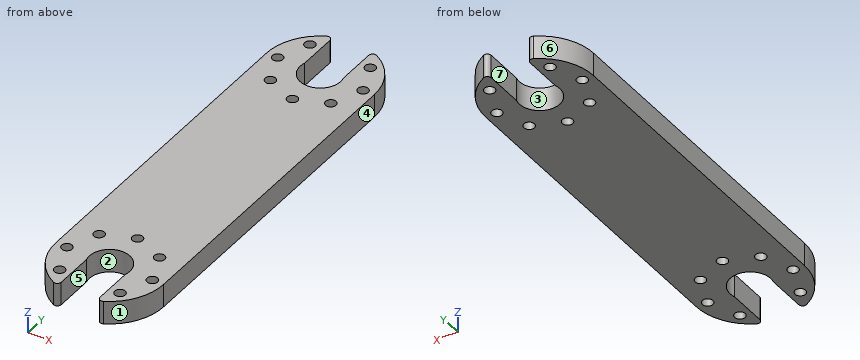
Autodesk Inventor part; units mm, degrees
ref_plane "YZ Plane" through (0, 0, 0) normal (1, 0, 0) x (0, 1, 0)
ref_plane "XZ Plane" through (0, 0, 0) normal (0, 1, 0) x (-1, 0, 0)
ref_plane "XY Plane" through (0, 0, 0) normal (0, 0, 1) x (1, 0, 0)
sketch "스케치1" plane through (0, 0, 0) normal (0, 0, 1) x (1, 0, 0)
  circle A0 centre (4.8832, 36.8726) radius 5
  circle A1 centre (4.8832, 47.8726) radius 1.55
  circle A2 centre (4.8832, 36.8726) radius 5
  arc A3 (-0.1168, 38.3009) -> (9.8832, 38.3009) centre (4.8832, 36.8726) ccw
  line L0 (4.8832, 42.0726) -> (9.8832, 42.0726)
  line L1 (4.8832, 42.0726) -> (-0.1168, 42.0726)
  circle A4 centre (4.8832, 36.8726) radius 13.9
  line L2 (9.8832, 42.0726) -> (9.8832, 49.8422)
  line L3 (-0.1168, 42.0726) -> (-0.1168, 49.8422)
  line L4 (9.8832, 42.0726) -> (9.8832, 38.3009)
  line L5 (-0.1168, 42.0726) -> (-0.1168, 38.3009)
  circle A5 centre (4.8832, 36.8726) radius 1.5
  line L6 (18.7832, 36.8726) -> (18.7832, -4.6274)
  line L7 (-9.0168, 36.8726) -> (-9.0168, -4.6274)
  arc A6 (-0.1168, 49.8422) -> (-9.0168, 36.8726) centre (4.8832, 36.8726) ccw
  arc A7 (18.7832, 36.8726) -> (9.8832, 49.8422) centre (4.8832, 36.8726) ccw
  line L8 (-9.0168, -4.6274) -> (18.7832, -4.6274)
  circle A8 centre (4.8832, 36.8726) radius 13.9
  line L9 (-9.0168, -46.1274) -> (-9.0168, -4.6274)
  line L10 (18.7832, -46.1274) -> (18.7832, -4.6274)
  line L11 (18.7832, -4.6274) -> (-9.0168, -4.6274)
  circle A9 centre (-2.895, 44.6508) radius 1.35
  circle A10 centre (-6.1168, 36.8726) radius 1.35
  circle A11 centre (-2.895, 29.0945) radius 1.35
  circle A12 centre (4.8832, 25.8726) radius 1.35
  circle A13 centre (12.6614, 29.0945) radius 1.35
  circle A14 centre (15.8832, 36.8726) radius 1.35
  circle A15 centre (12.6614, 44.6508) radius 1.35
  circle A16 centre (4.8832, -46.1274) radius 5
  circle A17 centre (4.8832, -57.1274) radius 1.55
  circle A18 centre (4.8832, -46.1274) radius 5
  arc A19 (9.8832, -47.5556) -> (-0.1168, -47.5556) centre (4.8832, -46.1274) ccw
  line L12 (4.8832, -51.3274) -> (-0.1168, -51.3274)
  line L13 (4.8832, -51.3274) -> (9.8832, -51.3274)
  line L14 (-0.1168, -51.3274) -> (-0.1168, -59.0969)
  line L15 (9.8832, -51.3274) -> (9.8832, -59.0969)
  line L16 (-0.1168, -51.3274) -> (-0.1168, -47.5556)
  line L17 (9.8832, -51.3274) -> (9.8832, -47.5556)
  circle A20 centre (4.8832, -46.1274) radius 1.5
  circle A21 centre (12.6614, -53.9055) radius 1.35
  circle A22 centre (15.8832, -46.1274) radius 1.35
  circle A23 centre (12.6614, -38.3492) radius 1.35
  circle A24 centre (4.8832, -35.1274) radius 1.35
  circle A25 centre (-2.895, -38.3492) radius 1.35
  circle A26 centre (-6.1168, -46.1274) radius 1.35
  circle A27 centre (-2.895, -53.9055) radius 1.35
  circle A28 centre (4.8832, -46.1274) radius 13.9
  point P0 (0, 0)
  point P1 (18.7832, -4.6274)
  point P2 (18.7832, -46.1274)
  dimension "d0" = 0.2
  dimension "d8" = 41.5
  dimension "d9" = 41.5
  dimension "d13" = 41.5
  dimension "d14" = 41.5
  dimension "d15" = 2.7
  dimension "d16" = 2.7
  dimension "d17" = 2.7
  dimension "d18" = 2.7
  dimension "d19" = 2.7
  dimension "d20" = 2.7
  dimension "d21" = 2.7
  dimension "d24" = 0.2
  dimension "d25" = 2.7
  dimension "d26" = 2.7
  dimension "d27" = 2.7
  dimension "d28" = 2.7
  dimension "d29" = 2.7
  dimension "d30" = 2.7
  dimension "d31" = 2.7
  dimension "d32" = 27.8
extrude "돌출1" add sketch "스케치1" along normal blind 6 contours A3 L4 L2 A4 L3 L5 | A4 L6 L8 L7 | L8 L10 A28 L9 | A28 L15 L17 A19 L16 L14
fillet "모깎기1" radius 1 4 edges at (-0.1168, 49.8422, 3) (9.8832, 49.8422, 3) (-0.1168, -59.0969, 3) (9.8832, -59.0969, 3)
properties part number "frame_ankle_to_knee1" material "PMMA 플라스틱"
Can you work these out from the model? Positions are in its coordinate system, mm. Face numbers are marked on the shaded views. A direction names the side the tool comes from. Coordinates: 2 decimals unless noted, no trailing zeros. Loops run counter-clockwise (first coordinate to the right, second up) from the corner with the lowest first, then second, coordinate; pieces in that order, holes last. Notation, with made-up numbers: (-17, 27) -> (-13, 27) arc R30 cw to (-13, 55) -> close; hole circle Ø1 at (84, 83). An arc over 180 degrees is marked (long way). Put each result on its own line as item: value. Start each with the question number.
Q1. I want a section at C-C (y = 41.5). Write out the boundary of the cut face in (x, z), plus the area to 3 significant figures.
Q2. I'm going to push flat-ended pins straight in: P1, Ø2.5, axis at x = 15.88, y = -46.13, coming from the +Z side; P2, Ø3, axis at y = 44, z = 1.5, coming from the -X side. Where does each tip first touch, or does it pass through?
Q3. For the marked faces 5, 6 and 7, which set-ups out of +Z, -Z, +X, -X, +Y, -Y let a thin tool reach every point of the face, with its end or its side?
Q4. Thinking about a two-plate mould opening in Y: for the marked faces 1, 2, 3 and 4, which applies, pulls with the +Y half, pulls with the -Y half, needs draft (parallel to the pull), parting line crosses it, or undercut?
Q5. If I drill on line 1 (Y direction, x = 11.5, z = 5.45); line 2 (Y direction, x = 4, z = 4.8); line 3 (Y direction, x = -7, z = 1.85), over which ranges is the centre line in solid material (lowest first)? Write a range as [from, to].
Q6. I want a section at B-B (x = -6.5). Write out the boundary of the cut face in (y, z), plus the area to 3 significant figures.
Q7. I want a section at A-A (z = 3.1). Count the separate pieces of the cut face and the enclosed holes in it, plus the area to 3 significant figures.
Taken from the geometry:
1. outline: (-8.22, 0) -> (-0.12, 0) -> (-0.12, 6) -> (-8.22, 6) -> close; (9.88, 0) -> (17.99, 0) -> (17.99, 6) -> (9.88, 6) -> close
1. area: 97.3 mm2
2. P1: passes through
2. P2: stops at x = -7.83
3. face 5: +Z, -Z, -Y
3. face 6: +Z, -Z, -X, +Y
3. face 7: +Z, -Z, +Y
4. face 1: pulls with the -Y half
4. face 2: undercut
4. face 3: undercut
4. face 4: needs draft
5. line 1: y = [-58.35, -54.59], [-53.22, -39.04], [-37.66, 28.41], [29.78, 43.96], [45.34, 49.1]
5. line 2: y = [-41, -36.15], [-34.11, 24.85], [26.89, 31.75]
5. line 3: y = [-53.34, -47.15], [-45.11, 35.85], [37.89, 44.08]
6. outline: (-54.1, 0) -> (-47.42, 0) -> (-47.42, 6) -> (-54.1, 6) -> close; (-44.83, 0) -> (35.58, 0) -> (35.58, 6) -> (-44.83, 6) -> close; (38.17, 0) -> (44.85, 0) -> (44.85, 6) -> (38.17, 6) -> close
6. area: 563 mm2
7. separate pieces: 1
7. enclosed holes: 14
7. area: 2,470 mm2
